from build123d import *


with BuildPart() as part:
    # Sketch1 → Revolve1 (revolve)
    with BuildSketch(Plane(origin=(0, 0, 0), x_dir=(0, 0, -1), z_dir=(1, 0, 0)), mode=Mode.PRIVATE) as revolve1_sk:
        Polygon((-184.976381406, 6.35), (91.883618594, 6.35), (91.883618594, 6.858), (94.423618594, 6.858), (94.423618594, 7.366), (90.677118594, 11.1125), (77.913618594, 11.1125), (76.135618594, 9.3345), (74.357618594, 11.1125), (-184.976381406, 11.1125), align=None)
    revolve(revolve1_sk.sketch.rotate(Axis((0, 0, 90.130122331), (0, 0, -1)), 90), axis=Axis((0, 0, 90.130122331), (0, 0, -1)))  # turned: the seam where the file's is


solid = part.part
CAD build for the part. Positions are in the model's coordinates, mm. A direction names the side the tool comes from. Give positions to 0.01 mm unless a question says otherwise; leave off trailing zeros. Write each loop counter-clockwise with the first axis right and the second up, starting at its lowest first coordinate (ties: lowest second). Pieces come first, ordered by that corner, then holes. Notation, with made-up numbers: (-24, 2) -> (-9, 2) arc R17 ccw to (-9, 15) -> close; hole circle Ø6 at (-15.75, 0). An arc over 180 degrees is marked (long way). Return JSON: item names as keys, results as strings.
Item 1: Tool access for faces 1 (the conical face through (9.01, -2.837, -76.024)), 2 (the flat face through (5, 5, 184.976)): list every direction of +Z, -Z, +X, -X, +Y, -Y with a clear straight run to the whole face (end or side of a thin tool).
Answer below:
{"face 1": "none", "face 2": "+Z, +X, -X, +Y, -Y"}
Item 2: Drill centre lines: probe 1 along X at (y, z) = (4.75, 19); probe 2 along Y at (x, z) = (0, 98); probe 3 along Y at (x, z) = (-3.5, -46.5). Where is each one in solid material? Low to high.
Answer below:
{"probe 1": "x = -10.05 to -4.21, 4.21 to 10.05", "probe 2": "y = -11.11 to -6.35, 6.35 to 11.11", "probe 3": "y = -10.55 to -5.3, 5.3 to 10.55"}
Item 3: Two-plate mould, pull along Y, no slides. Class faces 3 (the flat face through (-5, 5, -94.424)), 4 (the cylindrical face through (-8.2, -7.5, -84.2)), 5 (the cylindrical face through (-5.04, 3.86, 44.61)), 6 (the cylindrical face through (-1.487, 6.695, -93.171)): +Y half, -Y half, draft (parallel to the pull), parting line (faces both ways), or undercut.
Answer below:
{"face 3": "draft", "face 4": "parting line", "face 5": "undercut", "face 6": "undercut"}
Item 4: Drop flat-ended pins along their axis: pin 1 (1.5 mm diameter, centred on x = 1.5, y = 5, fed in from +Z); pin 2 (12 mm diameter, centred on x = 4, y = -0.5, fed in from +Z); pin 3 (4 mm diameter, centred on x = 5.5, z = 26, fed in from -Y); pin 4 (2 mm diameter, centred on y = 8.5, z = -11, fed in from -X). Give the stop position or say it passes through.
Answer below:
{"pin 1": "passes through", "pin 2": "stops at z = 184.98", "pin 3": "stops at y = -10.55", "pin 4": "stops at x = -8.2"}
Item 5: Band-saw the part on B-B (x = 0). List the corners of the cut face in (y, z), then the cut area to 3 significant figures.
Answer below:
{"outline": "(-11.11, -90.68) -> (-7.37, -94.42) -> (-6.86, -94.42) -> (-6.86, -91.88) -> (-6.35, -91.88) -> (-6.35, 184.98) -> (-11.11, 184.98) -> (-11.11, -74.36) -> (-9.33, -76.14) -> (-11.11, -77.91) -> close; (6.35, -91.88) -> (6.86, -91.88) -> (6.86, -94.42) -> (7.37, -94.42) -> (11.11, -90.68) -> (11.11, -77.91) -> (9.33, -76.14) -> (11.11, -74.36) -> (11.11, 184.98) -> (6.35, 184.98) -> close", "area": "2,640 mm2"}
